Autodesk Inventor part; units mm, degrees
ref_plane "YZ Plane" through (0, 0, 0) normal (1, 0, 0) x (0, 1, 0)
ref_plane "XZ Plane" through (0, 0, 0) normal (0, 1, 0) x (-1, 0, 0)
ref_plane "XY Plane" through (0, 0, 0) normal (0, 0, 1) x (1, 0, 0)
sketch "スケッチ1" plane through (0, 0, 0) normal (0, 1, 0) x (-1, 0, 0)
  line L0 (17, 7) -> (-17, 7)
  line L1 (-17, 7) -> (-17, -7)
  line L2 (-17, -7) -> (17, -7)
  line L3 (17, -7) -> (17, 7)
  line L4 (17, 7) -> (-17, -7) construction
  line L5 (-17, 7) -> (17, -7) construction
  point P0 (0, 0)
  dimension "d0" = 34
  dimension "d1" = 14
extrude "押し出し1" add sketch "スケッチ1" along normal blind 2.2
sketch "スケッチ2" plane through (0, 2.2, 0) normal (0, 1, 0) x (1, 0, 0)
  circle A0 centre (-10, 0) radius 5
  circle A1 centre (10, 0) radius 5
  point P0 (0, 0)
  dimension "d4" = 10
  dimension "d5" = 10
  dimension "d6" = 10
  dimension "d7" = 10
extrude "押し出し2" add sketch "スケッチ2" along normal blind 0.5
sketch "スケッチ3" plane through (-10, 2.7, 0) normal (0, 1, 0) x (1, 0, 0)
  circle A0 centre (0, 0) radius 5
  circle A1 centre (20, 0) radius 5
  circle A2 centre (0, 0) radius 3.95
  circle A3 centre (20, 0) radius 3.95
  point P0 (10, 0)
  dimension "d10" = 7.9
  dimension "d11" = 7.9
extrude "押し出し3" add sketch "スケッチ3" along normal blind 12 contours A2 | A3
sketch "スケッチ5" plane through (-10, 14.7, 0) normal (0, 1, 0) x (1, 0, 0)
  circle A0 centre (0, 0) radius 3.95
  circle A1 centre (20, 0) radius 3.95
  point P0 (10, 0)
hole "穴2" at (10, 14.7, 0) at (-10, 14.7, 0) direction (0, -1, 0) diameter 5.3 end through all
chamfer "面取り2" distance 0.2 angle 45 2 edges at (-13.95, 14.7, 0) (6.05, 14.7, 0)
fillet "フィレット2" radius 2 4 edges at (17, 1.1, 7) (17, 1.1, -7) (-17, 1.1, 7) (-17, 1.1, -7)
equation "\"d5\" = d4"
equation "\"d10\" = d11"
properties part number "scara-base8" material "ABS プラスチック"
Source: CAD feature listing. Evaluate the final solid. Frame: model axes, mm. A direction names the side the tool comes from. Round coordinates to 2 decimals unless told otherwise and drop trailing zeros. Order: outer loops, then holes, each group sorted by start corner. A loop starts at its lowest first (then second) coordinate and runs counter-clockwise, first axis right, second up. Notation, with made-up numbers: (42, -13) - (60, -13) arc R16 cw to (60, 5) - close; hole circle Ø11 at (4, 8). An arc over 180 degrees is marked (long way). Use a Markdown table: item, result. Add a question column.
1. Section query A-A (z = 0). Give the number of separate pieces and of enclosed holes in the cut face, then the cut area to 4 significant figures.
2. Section query B-B (x = -10). Return the cut outline in (y, z), then the cut area to 4 significant figures.
3. First-contact query: pin 1 (6 mm diameter, centred on y = 13, z = -2.5, fed in from +X); pin 2 (1 mm diameter, centred on x = 8, y = 11, fed in from -Z); pin 3 (1 mm diameter, centred on x = 4, z = -2, fed in from +Y). Flat tips, straight axial feed; report the tip coordinate or a pass-through.
4. Line query: probe 1 along X at (y, z) = (9.75, 0); probe 2 along Z at (x, y) = (10, 11); probe 3 along X at (y, z) = (13.75, 0.75). Output: solid intervals per line, ascending.
5. Set-up query: faces 1 (the cylindrical face through (14.77, 2.45, 1.5)), 2 (the cylindrical face through (-7.41, 7.25, -0.57)). Return all of +Z, -Z, +X, -X, +Y, -Y with unobstructed straight access to the full face (end or side cutting, diameter ignored); none if empty.
6. Section query C-C (y = 6). Return the cut outline in (x, z), then the cut area to 3 significant figures.
7. Section query D-D (z = 4.5). Return the cut outline in (x, y), then the cut area to 3 significant figures.
8. Mould query, pull axis X, two halves, no side actions, for faces 3 (the flat face through (14, 2.7, -2)), 4 (the flat face through (0, 1, 7)), 5 (the flat face through (0, 2.2, 0)), 6 (the flat face through (-17, 1, 0)). Classes: +X half, -X half, draft (parallel to the pull), parting line (faces both ways), or undercut.
Derived:
| question | item | result |
|---|---|---|
| 1 | separate pieces | 3 |
| 1 | enclosed holes | 0 |
| 1 | area | 118.5 mm2 |
| 2 | outline | (0, -7) - (2.2, -7) - (2.2, -5) - (2.7, -5) - (2.7, -3.95) - (14.5, -3.95) - (14.7, -3.75) - (14.7, -2.65) - (0, -2.65) - close; (0, 2.65) - (14.7, 2.65) - (14.7, 3.75) - (14.5, 3.95) - (2.7, 3.95) - (2.7, 5) - (2.2, 5) - (2.2, 7) - (0, 7) - close |
| 2 | area | 52.65 mm2 |
| 3 | pin 1 | x = 13.95 |
| 3 | pin 2 | z = -3.65 |
| 3 | pin 3 | y = 2.2 |
| 4 | probe 1 | -13.95 to -12.65, -7.35 to -6.05, 6.05 to 7.35, 12.65 to 13.95 |
| 4 | probe 2 | -3.95 to -2.65, 2.65 to 3.95 |
| 4 | probe 3 | -13.88 to -12.54, -7.46 to -6.12, 6.12 to 7.46, 12.54 to 13.88 |
| 5 | face 1 | +Y |
| 5 | face 2 | +Y, -Y |
| 6 | outline | circle Ø7.9 at (-10, 0); circle Ø7.9 at (10, 0); hole circle Ø5.3 at (-10, 0); hole circle Ø5.3 at (10, 0) |
| 6 | area | 53.9 mm2 |
| 7 | outline | (-17, 0) - (17, 0) - (17, 2.2) - (12.18, 2.2) - (12.18, 2.7) - (7.82, 2.7) - (7.82, 2.2) - (-7.82, 2.2) - (-7.82, 2.7) - (-12.18, 2.7) - (-12.18, 2.2) - (-17, 2.2) - close |
| 7 | area | 79.2 mm2 |
| 8 | face 3 | undercut |
| 8 | face 4 | draft |
| 8 | face 5 | undercut |
| 8 | face 6 | -X half |
